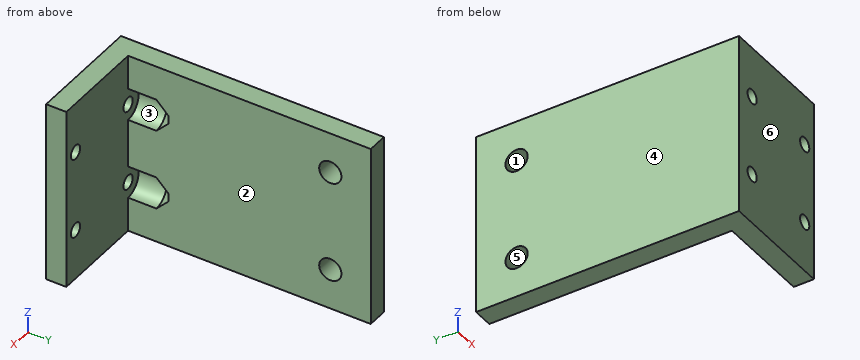
from build123d import *

# Parameters (mm, degrees)
BOSS_EXTRU_1_DEPTH      = 45
ENL_V_MAT_EXTRU_1_REACH = 83.904
ESQUISSE2_R             = 1.75
ENL_V_MAT_EXTRU_2_REACH = 86.037
ESQUISSE3_R             = 2.75
ESQUISSE4_R             = 4
ENL_V_MAT_EXTRU_3_DEPTH = 10
CHANFREIN1_SIZE         = 3


with BuildPart() as part:
    # Esquisse1 → Boss.-Extru.1 (new body)
    with BuildSketch(Plane.XY):
        Polygon((-32.913141208, 0), (-4.413141208, 0), (-4.413141208, 5), (-27.913141208, 5), (-27.913141208, 65), (-32.913141208, 65), align=None)
    extrude(amount=BOSS_EXTRU_1_DEPTH)

    # Esquisse2 → Enlèv. mat.-Extru.1 (cut, up to next)
    with BuildSketch(Plane(origin=(0, 5, 0), x_dir=(1, 0, 0), z_dir=(0, 1, 0)), mode=Mode.PRIVATE) as enl_v_mat_extru_1_sk1:
        with Locations(Location((-27.913141208, -32.5, 0), (0, 0, 270))):
            Circle(ESQUISSE2_R)
    enl_v_mat_extru_1_tool1 = extrude(enl_v_mat_extru_1_sk1.sketch, amount=-ENL_V_MAT_EXTRU_1_REACH, mode=Mode.PRIVATE) & part.part
    # Esquisse2 → Enlèv. mat.-Extru.1 (cut, up to next)
    with BuildSketch(Plane(origin=(0, 5, 0), x_dir=(1, 0, 0), z_dir=(0, 1, 0)), mode=Mode.PRIVATE) as enl_v_mat_extru_1_sk2:
        with Locations(Location((-27.913141208, -12.5, 0), (0, 0, 270))):
            Circle(ESQUISSE2_R)
    enl_v_mat_extru_1_tool2 = extrude(enl_v_mat_extru_1_sk2.sketch, amount=-ENL_V_MAT_EXTRU_1_REACH, mode=Mode.PRIVATE) & part.part
    # Esquisse2 → Enlèv. mat.-Extru.1 (cut, up to next)
    with BuildSketch(Plane(origin=(0, 5, 0), x_dir=(1, 0, 0), z_dir=(0, 1, 0)), mode=Mode.PRIVATE) as enl_v_mat_extru_1_sk3:
        with Locations(Location((-7.913141208, -12.5, 0), (0, 0, 180))):
            Circle(ESQUISSE2_R)
    enl_v_mat_extru_1_tool3 = extrude(enl_v_mat_extru_1_sk3.sketch, amount=-ENL_V_MAT_EXTRU_1_REACH, mode=Mode.PRIVATE) & part.part
    # Esquisse2 → Enlèv. mat.-Extru.1 (cut, up to next)
    with BuildSketch(Plane(origin=(0, 5, 0), x_dir=(1, 0, 0), z_dir=(0, 1, 0)), mode=Mode.PRIVATE) as enl_v_mat_extru_1_sk4:
        with Locations(Location((-7.913141208, -32.5, 0), (0, 0, 180))):
            Circle(ESQUISSE2_R)
    enl_v_mat_extru_1_tool4 = extrude(enl_v_mat_extru_1_sk4.sketch, amount=-ENL_V_MAT_EXTRU_1_REACH, mode=Mode.PRIVATE) & part.part
    add(enl_v_mat_extru_1_tool1.solids().sort_by_distance((-27.913141, 5, 32.5))[0], mode=Mode.SUBTRACT)
    add(enl_v_mat_extru_1_tool2.solids().sort_by_distance((-27.913141, 5, 12.5))[0], mode=Mode.SUBTRACT)
    add(enl_v_mat_extru_1_tool3.solids().sort_by_distance((-7.913141, 5, 12.5))[0], mode=Mode.SUBTRACT)
    add(enl_v_mat_extru_1_tool4.solids().sort_by_distance((-7.913141, 5, 32.5))[0], mode=Mode.SUBTRACT)

    # Esquisse3 → Enlèv. mat.-Extru.2 (cut, up to next)
    with BuildSketch(Plane.ZY.offset(32.913141208), mode=Mode.PRIVATE) as enl_v_mat_extru_2_sk1:
        with Locations(Location((10, 55, 0), (0, 0, 270))):
            Circle(ESQUISSE3_R)
    enl_v_mat_extru_2_tool1 = extrude(enl_v_mat_extru_2_sk1.sketch, amount=-ENL_V_MAT_EXTRU_2_REACH, mode=Mode.PRIVATE) & part.part
    # Esquisse3 → Enlèv. mat.-Extru.2 (cut, up to next)
    with BuildSketch(Plane.ZY.offset(32.913141208), mode=Mode.PRIVATE) as enl_v_mat_extru_2_sk2:
        with Locations(Location((35, 55, 0), (0, 0, 270))):
            Circle(ESQUISSE3_R)
    enl_v_mat_extru_2_tool2 = extrude(enl_v_mat_extru_2_sk2.sketch, amount=-ENL_V_MAT_EXTRU_2_REACH, mode=Mode.PRIVATE) & part.part
    add(enl_v_mat_extru_2_tool1.solids().sort_by_distance((-32.913141, 55, 10))[0], mode=Mode.SUBTRACT)
    add(enl_v_mat_extru_2_tool2.solids().sort_by_distance((-32.913141, 55, 35))[0], mode=Mode.SUBTRACT)

    # Esquisse4 → Enlèv. mat.-Extru.3 (cut)
    with BuildSketch(Plane(origin=(0, 5, 0), x_dir=(1, 0, 0), z_dir=(0, 1, 0))):
        with Locations((-27.913141208, -32.5)):
            Circle(ESQUISSE4_R)
        with Locations((-27.913141208, -12.5)):
            Circle(ESQUISSE4_R)
    extrude(amount=ENL_V_MAT_EXTRU_3_DEPTH, mode=Mode.SUBTRACT)

    # Chanfrein1
    chanfrein1_edges = [part.edges().sort_by_distance(p)[0] for p in [
        (-31.913141208, 15, 32.5),
        (-31.913141208, 15, 12.5),
    ]]
    chamfer(chanfrein1_edges, length=CHANFREIN1_SIZE)


solid = part.part
Input: part model. Units: mm. Frame: model coordinates. Face numbers are marked on the shaded views. A direction names the side the tool comes from. Give positions to 0.01 mm unless a question says otherwise; leave off trailing zeros. Order: outer loops, then holes, each group sorted by start corner. A loop starts at its lowest first (then second) coordinate and runs counter-clockwise, first axis right, second up. Notation, with made-up numbers: (-11.5, 13.25) - (29.5, 13.25) arc R28 cw to (29.5, 32.25) - close; hole circle Ø9 at (-5.5, 6). An arc over 180 degrees is marked (long way). Write each question's results on one line, items separated by ' | '.
Item 1: Section B-B (y = 4). Return loops of the section in (x, z).
A:
outline: (-32.91, 0) - (-4.41, 0) - (-4.41, 45) - (-32.91, 45) - close; hole circle Ø3.5 at (-27.91, 12.5); hole circle Ø3.5 at (-27.91, 32.5); hole circle Ø3.5 at (-7.91, 12.5); hole circle Ø3.5 at (-7.91, 32.5)
Item 2: Section D-D (z = 26). Return loops of the section in (x, y).
A:
outline: (-32.91, 0) - (-4.41, 0) - (-4.41, 5) - (-27.91, 5) - (-27.91, 65) - (-32.91, 65) - close
Item 3: Draft query along Y for the marked faces 4, 5 and 6. Return one class per face: released by +Y, released by -Y, zero draft, split by the parting line, or undercut.
A:
face 4: zero draft | face 5: undercut | face 6: released by -Y
Item 4: Section A-A (y = 55). Return loops of the section in (x, z).
A:
outline: (-32.91, 0) - (-27.91, 0) - (-27.91, 7.25) - (-32.91, 7.25) - close; (-32.91, 12.75) - (-27.91, 12.75) - (-27.91, 32.25) - (-32.91, 32.25) - close; (-32.91, 37.75) - (-27.91, 37.75) - (-27.91, 45) - (-32.91, 45) - close
Item 5: Material intervals for line 1 along Y through (x, z) = (-27.25, 27); line 2 along X through (y, z) = (22, 25.5); line 3 along X through (y, z) = (2, 32), sorted ascending.
A:
line 1: y = 0 to 5 | line 2: x = -32.91 to -27.91 | line 3: x = -32.91 to -29.59, -26.24 to -9.59, -6.24 to -4.41
Item 6: Contact query for flat-ended pins moving along their axis: pin 1 Ø0.5 at (x, z) = (-28, 32) entering from -Y; pin 2 Ø22.5 at (y, z) = (34, 13.5) entering from +X; pin 3 Ø3 at (x, z) = (-27.91, 32.5) entering from -Y. Output: stop coordinate, or through.
A:
pin 1: stops at y = 15 | pin 2: stops at x = -27.91 | pin 3: stops at y = 14.5
Item 7: Section C-C (x = -7.5). Return loops of the section in (y, z).
A:
outline: (0, 0) - (5, 0) - (5, 10.8) - (0, 10.8) - close; (0, 14.2) - (5, 14.2) - (5, 30.8) - (0, 30.8) - close; (0, 34.2) - (5, 34.2) - (5, 45) - (0, 45) - close
Item 8: Access query for the marked faces 1, 2 and 3. Directions: +Z, -Z, +X, -X, +Y, -Y. A direction counts if a zero-diameter tool reaches every point of the face in a straight line with its end or side. Return the directions, or none.
A:
face 1: +X, -X | face 2: +Z, -Z, +X, +Y | face 3: +X
